from build123d import *

# Parameters (mm, degrees)
F0_R        = 63.5
F0_R_2      = 12.5
F1_DEPTH    = 20
F2_DEPTH    = 1060
F2_FACE_R   = 63.5
F2_FACE_R_2 = 12.5
F3_DEPTH    = 558.8


with BuildPart() as f1:
    # F0 (on Front) → F1 (new body)
    with BuildSketch(Plane.XZ):
        Circle(F0_R)
        Circle(F0_R_2, mode=Mode.SUBTRACT)
        Circle(F0_R_2)
    extrude(amount=F1_DEPTH)

    # F0 (on Front) → F2 (join)
    with BuildSketch(Plane.XZ):
        Circle(F0_R)
        Circle(F0_R_2, mode=Mode.SUBTRACT)
    extrude(amount=F2_DEPTH)

    # F0 (on Front) + F2_face (on face) → F3 (join)
    with BuildSketch(Plane.XZ):
        Circle(F0_R)
        Circle(F0_R_2, mode=Mode.SUBTRACT)
    with BuildSketch(Plane.XZ.offset(1060)):
        Circle(F2_FACE_R)
        Circle(F2_FACE_R_2, mode=Mode.SUBTRACT)
    extrude(amount=-F3_DEPTH)


solid = f1.part
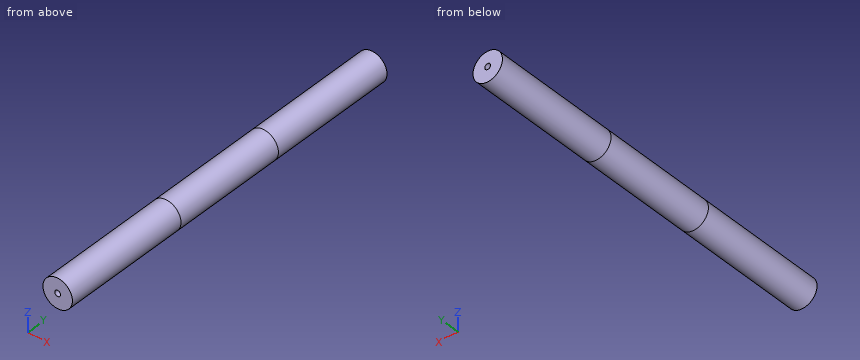
Input: part model. Units: mm. Frame: model coordinates. Give positions to 0.01 mm unless a question says otherwise; leave off trailing zeros. Write each loop counter-clockwise with the first axis right and the second up, starting at its lowest first coordinate (ties: lowest second). Pieces come first, ordered by that corner, then holes.
Q1. Material intervals for probe 1 along Z at (x, y) = (0, -850); probe 2 along Y at (x, z) = (3.5, -8); probe 3 along X at (y, z) = (-940.5, 54.5), sorted ascending.
Q2. Section A-A, the plane y = -961. Output: boundary loops of the cut face in (x, z).
Q3. Section C-C, the plane z = -38.5. Output: boundary loops of the cut face in (x, y).
Q4. First-contact query: P1, Ø3, axis at x = 15.5, y = -732.5, coming from the +Z side; P2, Ø1, axis at x = -15, y = -467, coming from the +Z side; P3, Ø12, axis at y = 11.5, z = 33.5, coming from the -X side. Flat tips, straight axial feed; report the tip coordinate or a pass-through.
Q5. Section B-B, the plane z = 43.5. Output: boundary loops of the cut face in (x, y).
Filled in:
1. probe 1: z = -63.5 to -12.5, 12.5 to 63.5
1. probe 2: y = -20 to 0
1. probe 3: x = -32.59 to 32.59
2. outline: circle Ø127 at (0, 0); hole circle Ø25 at (0, 0)
3. outline: (-50.5, -1060) - (50.5, -1060) - (50.5, 558.8) - (-50.5, 558.8) - close
4. P1: stops at z = 61.94
4. P2: stops at z = 61.82
4. P3: stops at x = -57.24
5. outline: (-46.26, -1060) - (46.26, -1060) - (46.26, 558.8) - (-46.26, 558.8) - close
